Can you work these out from the model? Positions are in its coordinate system, mm. Give positions to 0.01 mm unless a question says otherwise; leave off trailing zeros. Loops run counter-clockwise (first coordinate to the right, second up) from the corner with the lowest first, then second, coordinate; pieces in that order, holes last. Notation, with made-up numbers: M -17,10.25 L -13,10.25 A18 ccw -13,19.25 Z; hole C 10,24.25 d6. An arc over 180 degrees is marked long. Put each result on its own line as item: value. Start each with the question number.
1) Please list where these lines run through material, in increasing order: line 1 along X through (y, z) = (3, 0.3); line 2 along Y through (x, z) = (-3, 0.55); line 3 along X through (y, z) = (1.75, 0.55). Write a range as from..to.
2) Imagine slicing it at C-C (y = 2.5). Write out the boundary of the cut face in (x, z), then the cut area to 3 significant figures.
3) Imagine slicing it at A-A (z = 0.25). Write out the boundary of the cut face in (x, y), then the cut area to 3 significant figures.
4) Imagine slicing it at B-B (x = -3). Write out the boundary of the cut face in (y, z).
from build123d import *

# Parameters (mm, degrees)
F0_W     = 6.2
F0_H     = 7
F2_DEPTH = 0.6
F4_R     = 0.5


with BuildPart() as f2:
    # F1 (on Top) + F0 (on Top) → F2 (new body)
    with BuildSketch(Plane.XY):
        Polygon((1.025447, 3.5), (0, 3.5), (-1.025447, 3.5), (-3.75, 1.585766), (-3.75, 0), (-3.75, -1.585766), (-1.025447, -3.5), (0, -3.5), (1.025447, -3.5), (3.75, -1.585766), (3.75, 0), (3.75, 1.585766), align=None)
    with BuildSketch(Plane.XY):
        Rectangle(F0_W, F0_H)
    extrude(amount=F2_DEPTH)

    # F3: union 

    # F4
    f4_edges = [f2.edges().sort_by_distance(p)[0] for p in [
        (-3.1, 3.5, 0.3),
        (-3.1, -3.5, 0.3),
        (3.1, -3.5, 0.3),
        (3.1, 3.5, 0.3),
    ]]
    fillet(f4_edges, radius=F4_R)


solid = f2.part
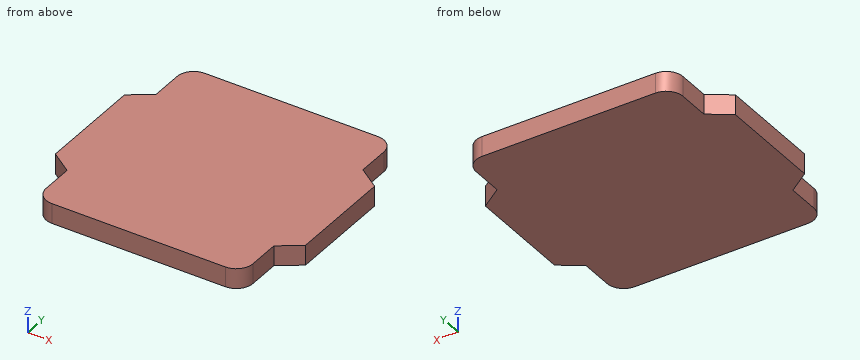
Recorded:
1. line 1: -3.1..3.1
1. line 2: -3.3..3.3
1. line 3: -3.52..3.52
2. outline: M -3.1,0 L 3.1,0 L 3.1,0.6 L -3.1,0.6 Z
2. area: 3.72 mm²
3. outline: M -3.75,-1.59 L -3.1,-2.04 L -3.1,-3 A0.5 ccw -2.6,-3.5 L 2.6,-3.5 A0.5 ccw 3.1,-3 L 3.1,-2.04 L 3.75,-1.59 L 3.75,1.59 L 3.1,2.04 L 3.1,3 A0.5 ccw 2.6,3.5 L -2.6,3.5 A0.5 ccw -3.1,3 L -3.1,2.04 L -3.75,1.59 Z
3. area: 47.9 mm²
4. outline: M -3.3,0 L 3.3,0 L 3.3,0.6 L -3.3,0.6 Z
